from build123d import *

# Parameters (mm, degrees)
F1_DEPTH = 22
F2_R     = 10
F3_R     = 3
F4_R     = 4
F5_R     = 5
F6_R     = 2
F7_R     = 2


with BuildPart() as f1:
    # F0 (on Top) → F1 (new body)
    with BuildSketch(Plane.XY):
        with BuildLine():
            ThreePointArc((-43.69757, 0), (-26.876888, -25.571939), (-23.561389, -56))
            Line((-23.561389, -56), (-7.5, -56))
            Line((-7.5, -56), (-7.5, -50))
            Line((-7.5, -50), (-11, -50))
            Line((-11, -50), (-11, -20))
            Line((-11, -20), (-5, -20))
            Line((-5, -20), (-5, -25))
            Line((-5, -25), (0, -25))
            Line((0, -25), (0, 0))
            Line((0, 0), (0, 10))
            Line((0, 10), (-12, 10))
            Line((-12, 10), (-12, 6))
            Line((-12, 6), (-72, 6))
            Line((-72, 6), (-72, 10))
            Line((-72, 10), (-76, 10))
            Line((-76, 10), (-76, 0))
            Line((-76, 0), (-43.69757, 0))
        make_face()
        with BuildLine():
            Line((-6, -14), (-25.474719, -14))
            ThreePointArc((-25.474719, -14), (-29.967584, -6.70409), (-35.303435, 0))
            Line((-35.303435, 0), (-6, 0))
            Line((-6, 0), (-6, -14))
        make_face(mode=Mode.SUBTRACT)
    extrude(amount=F1_DEPTH)

    # F2
    f2_edges = [f1.edges().sort_by_distance(p)[0] for p in [
        (-43.69757, 0, 11),
    ]]
    fillet(f2_edges, radius=F2_R)

    # F3
    f3_edges = [f1.edges().sort_by_distance(p)[0] for p in [
        (-23.561389, -56, 11),
    ]]
    fillet(f3_edges, radius=F3_R)

    # F4
    f4_edges = [f1.edges().sort_by_distance(p)[0] for p in [
        (-35.303435, 0, 11),
        (-6, 0, 11),
        (-25.474719, -14, 11),
        (-6, -14, 11),
    ]]
    fillet(f4_edges, radius=F4_R)

    # F5
    f5_edges = [f1.edges().sort_by_distance(p)[0] for p in [
        (0, 10, 11),
    ]]
    fillet(f5_edges, radius=F5_R)

    # F6
    f6_edges = [f1.edges().sort_by_distance(p)[0] for p in [
        (-12, 6, 11),
        (-72, 6, 11),
    ]]
    fillet(f6_edges, radius=F6_R)

    # F7
    f7_edges = [f1.edges().sort_by_distance(p)[0] for p in [
        (-76, 10, 11),
        (-76, 0, 11),
    ]]
    fillet(f7_edges, radius=F7_R)


solid = f1.part
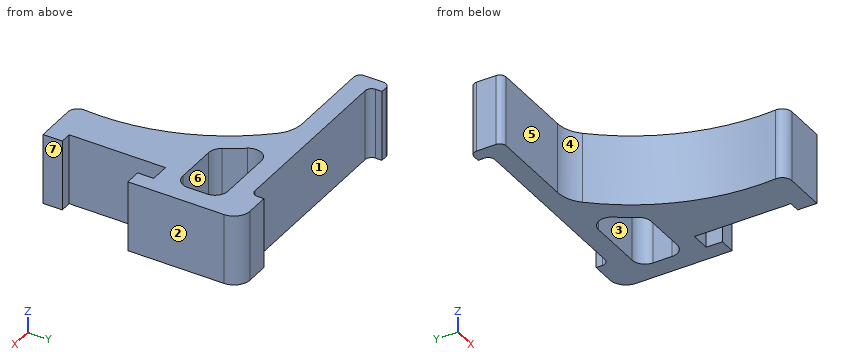
Geometry: final body of the model. Coordinates: model frame, mm. Face numbers are marked on the shaded views. A direction names the side the tool comes from. Give positions to 0.01 mm unless a question says otherwise; leave off trailing zeros. Write each loop counter-clockwise with the first axis right and the second up, starting at its lowest first coordinate (ties: lowest second). Pieces come first, ordered by that corner, then holes. Notation, with made-up numbers: M 44.25,68.25 L 58.25,68.25 A11 cw 58.25,77.25 Z; hole C 36,-8.75 d8. An arc over 180 degrees is marked long. Answer in a Markdown table with one row per item. Add a question column.
(1) Reachability of the marked faces 5, 6 and 7 from +Z, -Z, +X, -X, +Y, -Y: full face, straight path, thin tool, end or side. Return the list, or none.
(2) Section D-D on x = -50.5. Return loops of the section in (y, z).
(3) Ray query, line 1 (Y direction, x = -8, z = 15); line 2 (X direction, y = -24, z = 7.5); line 3 (Y direction, x = -15, z = 3.25). Return the intervals inside material, ascending.
(4) Mould query, pull axis Y, two halves, no side actions, for the marked faces 1, 2, 3 and 4. Classes: +Y half, -Y half, draft (parallel to the pull), parting line (faces both ways), or undercut.
(5) First-contact query: pin 1 (4 mm diameter, centred on x = -32, z = 16, fed in from +Y); pin 2 (4 mm diameter, centred on y = -21.5, z = 13.5, fed in from -X); pin 3 (6.5 mm diameter, centred on y = -6, z = 15, fed in from -X); pin 4 (12 mm diameter, centred on x = -22.5, z = 12.5, fed in from -Y). Flat tips, straight axial feed; report the tip coordinate or a pass-through.
(6) Section A-A on x = -15.5. Return loops of the section in (y, z).
(7) Section C-C on y = -24. Return loops of the section in (x, z), and give its area (3 significant figures).
Result set:
| question | item | result |
|---|---|---|
| 1 | face 5 | +Z, -Z, -X, -Y |
| 1 | face 6 | +Z, -Z |
| 1 | face 7 | +Z, -Z, +X, -Y |
| 2 | outline | M 0,0 L 6,0 L 6,22 L 0,22 Z |
| 3 | line 1 | y = -56 to -50, -20 to -13.46, -0.54 to 10 |
| 3 | line 2 | x = -27.47 to -11, -5 to 0 |
| 3 | line 3 | y = -56 to -14, 0 to 6 |
| 4 | face 1 | +Y half |
| 4 | face 2 | draft |
| 4 | face 3 | undercut |
| 4 | face 4 | -Y half |
| 5 | pin 1 | stops at y = 6 |
| 5 | pin 2 | stops at x = -29.41 |
| 5 | pin 3 | stops at x = -40.95 |
| 5 | pin 4 | stops at y = -56 |
| 6 | outline | M -56,0 L -14,0 L -14,22 L -56,22 Z; M 0,0 L 6,0 L 6,22 L 0,22 Z |
| 7 | outline | M -27.47,0 L -11,0 L -11,22 L -27.47,22 Z; M -5,0 L 0,0 L 0,22 L -5,22 Z |
| 7 | area | 472 mm^2 |
